Autodesk Inventor part; units mm, degrees
ref_plane "YZ Plane" through (0, 0, 0) normal (1, 0, 0) x (0, 1, 0)
ref_plane "XY Plane" through (0, 0, 0) normal (0, 0, 1) x (1, 0, 0)
sketch "Sketch1" plane through (0, 0, 0) normal (0, 0, 1) x (1, 0, 0)
  line L0 (0, -11) -> (-10.5, -11)
  line L1 (-10.5, -11) -> (-10.5, 31)
  line L2 (-10.5, 31) -> (10.5, 31)
  line L3 (10.5, 31) -> (10.5, -11)
  line L4 (10.5, -11) -> (0, -11)
  line L5 (10.5, 10) -> (0, 10)
  line L6 (0, 0) -> (0, 10)
  circle A0 centre (0, 0) radius 42.5
  dimension "d1" = 42
  dimension "d28" = 21
  dimension "d76" = 10
  dimension "d77" = 10.5
  dimension "d78" = 85
extrude "Extrusion6" add sketch "Sketch1" along normal blind 5
sketch "Sketch9" plane through (0, 0, 5) normal (0, 0, 1) x (1, 0, 0)
  line L0 (10.5, -11) -> (-10.5, -11)
  line L1 (0, -11) -> (0, -14)
  line L2 (0, -14) -> (-5, -14)
  circle A0 centre (-5, -14) radius 3
  line L3 (0, -14) -> (5, -14)
  circle A1 centre (5, -14) radius 3
  line L4 (-10.5, -11) -> (-10.5, 31)
  line L5 (-10.5, 10) -> (10.5, 10)
  line L6 (10.5, 31) -> (-10.5, 31)
  line L7 (0, 31) -> (0, 34)
  line L8 (0, 34) -> (-5, 34)
  circle A2 centre (-5, 34) radius 3
  line L9 (0, 34) -> (5, 34)
  circle A3 centre (5, 34) radius 3
  dimension "d79" = 3
  dimension "d80" = 5
  dimension "d81" = 6
  dimension "d82" = 5
  dimension "d83" = 6
extrude "Extrusion12" cut sketch "Sketch9" against normal through all contours A2 | A1 | A0 | A3
sketch "Sketch10" plane through (0, 0, 5) normal (0, 0, 1) x (1, 0, 0)
  line L0 (-10.5, 31) -> (-10.5, 38.5)
  circle A0 centre (0, 0) radius 39.9061
  line L1 (-10.5, -11) -> (-10.5, -18.5)
  arc A1 (-21.272, 0) -> (21.272, 0) centre (0, 0) ccw
  arc A2 (-21.272, 0) -> (-10.5, 31) centre (-71.284, 34.75) ccw
  line L2 (10.5, 31) -> (10.5, 38.5)
  arc A3 (10.5, 31) -> (21.272, 0) centre (71.284, 34.75) ccw
  dimension "d86" = 7.5
  dimension "d87" = 79.8123
  dimension "d88" = 7.5
extrude "Extrusion13" add sketch "Sketch10" along normal blind 35 contours A2 A1 A3 L2 A0 L0 picked at (-28.5299, 15.6602)
sketch "Sketch11" plane through (0, 0, 40) normal (0, 0, 1) x (1, 0, 0)
  line L0 (0, 0) -> (0, -30)
  circle A0 centre (0, -30) radius 1.75
  circle A1 centre (21.2132, -21.2132) radius 1.75
  circle A2 centre (30, 0) radius 1.75
  circle A3 centre (21.2132, 21.2132) radius 1.75
  circle A4 centre (0, 30) radius 1.75
  circle A5 centre (-21.2132, 21.2132) radius 1.75
  circle A6 centre (-30, 0) radius 1.75
  circle A7 centre (-21.2132, -21.2132) radius 1.75
  dimension "d91" = 30
  dimension "d92" = 3.5
  dimension "d95" = 360
extrude "Extrusion14" cut sketch "Sketch11" against normal through all contours A0 | A1 | A2 | A3 | A5 | A6 | A7
sketch "Sketch12" plane through (0, 0, 40) normal (0, 0, 1) x (1, 0, 0)
  line L0 (0, 0) -> (0, -39.9061)
  arc A0 (-10.5, 38.5) -> (10.5, 38.5) centre (0, 0) ccw
ref_plane "Work Plane2" through (0, -39.9061, 40) normal (0, 1, 0) x (-1, 0, 0)
sketch "Sketch13" plane through (0, -39.9061, 40) normal (0, 1, 0) x (-1, 0, 0)
  line L0 (-0.0018, 0) -> (-0.0018, -10)
  line L1 (-0.0018, -10) -> (-4.0018, -10)
  line L2 (-4.0018, -10) -> (-4.0018, -14)
  line L3 (-4.0018, -14) -> (3.9982, -14)
  line L4 (3.9982, -14) -> (3.9982, -10)
  line L5 (3.9982, -10) -> (-0.0018, -10)
  point P0 (0, -40)
  dimension "d99" = 10
  dimension "d100" = 4
  dimension "d101" = 4
  dimension "d102" = 8
extrude "Extrusion15" cut sketch "Sketch13" along normal blind 15
pattern_circular "Circular Pattern2" count 8 over 360 about axis through (0, 0, 5) along (0, 0, 1) of "Extrusion15"
properties part number "Base"
Build history of the part. All positions in model axes, mm. A direction names the side the tool comes from. Give positions to 0.01 mm unless a question says otherwise; leave off trailing zeros. Order: outer loops, then holes, each group sorted by start corner. A loop starts at its lowest first (then second) coordinate and runs counter-clockwise, first axis right, second up. Notation, with made-up numbers: M 88.5,1 L 109.5,1 A19 cw 109.5,37 Z; hole C -0.5,23 d3. An arc over 180 degrees is marked long. Write item = value, one per line. Start each with the question number.
(1) Which spindle directions (+Z, -Z, +X, -X, +Y, -Y) get a long thin tool onto all of the face, cutting with end or side? Do faces 4 (the flat face through (24.906, 0, 28)), 5 (the flat face through (25.75, -20.09, 28.03)), 6 (the flat face through (0, 32, 5)), 7 (the flat face through (-10.5, 10, 2)), 8 (the flat face through (-32, -4.002, 28)). Say none if no direction does.
(2) Two-plate mould, pull along Y, no slides. Class faces 1 (the flat face through (0, -24.906, 28)), 2 (the cylindrical face through (-22.96, 21.29, 35.07)), 3 (the flat face through (0, -33, 30)): released by +Y, released by -Y, zero draft, split by the parting line, or undercut.
(3) Probe L1, parallel to X at y = 0, z = 32.5; L2, parallel to Y at x = 0, z = 33; L3, parallel to Y at x = -22, z = 20.5. List the from-to ranges inside material, lowest first. Write a range as [from, to].
(4) Slice it at B-B on x = 0. Write the cut outline in (y, z), plus the area to 3 significant figures.
(5) Pin check, flat tips, straight feed: pin 1 Ø10 at (x, z) = (-15, 8) entering from -Y; pin 2 Ø10 at (y, z) = (0.5, 32.5) entering from -X; pin 3 Ø12 at (x, z) = (-12, 34.5) entering from +Y. Stop position of each tip, or through.
(6) Slice it at A-A on y = 16. Write the cut outline in (x, z).
(7) Slice it at C-C on z = 22. Write the cut outline in (x, y), plus the area to 3 significant figures.
Responses:
q1.face_4 = +X
q1.face_5 = none
q1.face_6 = +Z
q1.face_7 = +Z, -Z
q1.face_8 = -X
q2.face_1 = released by -Y
q2.face_2 = undercut
q2.face_3 = zero draft
q3.L1 = [-39.91, -31.75], [-28.25, -21.27], [21.27, 28.25], [31.75, 39.91]
q3.L2 = [-39.91, -31.75], [-28.25, -21.27]
q3.L3 = [-33.29, -22.78], [-19.65, 19.65], [22.78, 33.29]
q4.outline = M -42.5,0 L -31.75,0 L -31.75,26 L -39.91,26 L -39.91,5 L -42.5,5 Z; M -39.91,30 L -31.75,30 L -31.75,40 L -39.91,40 Z; M -28.25,0 L -11,0 L -11,5 L -21.27,5 L -21.27,40 L -28.25,40 L -28.25,30 L -24.91,30 L -24.91,26 L -28.25,26 Z; M 31,0 L 42.5,0 L 42.5,5 L 31,5 Z
q4.area = 681 mm2
q5.pin_1 = -41.05
q5.pin_2 = -39.91
q5.pin_3 = 38.5
q6.outline = M -39.37,0 L -10.5,0 L -10.5,5 L -13.34,5 L -13.34,40 L -36.56,40 L -36.56,5 L -39.37,5 Z; M 10.5,0 L 39.37,0 L 39.37,5 L 36.56,5 L 36.56,40 L 13.34,40 L 13.34,5 L 10.5,5 Z; hole M -21.66,26 L -19.22,26 L -19.22,30 L -21.66,30 Z; hole M 19.22,26 L 21.65,26 L 21.65,30 L 19.22,30 Z
q7.outline = M -21.27,0 A60.9 ccw -10.5,31 L -10.5,38.5 A39.91 ccw long 10.5,38.5 L 10.5,31 A60.9 ccw 21.27,0 A21.27 cw Z; hole C -30,0 d3.5; hole C -21.21,-21.21 d3.5; hole C -21.21,21.21 d3.5; hole C 0,-30 d3.5; hole C 21.21,-21.21 d3.5; hole C 21.21,21.21 d3.5; hole C 30,0 d3.5
q7.area = 3,160 mm2
